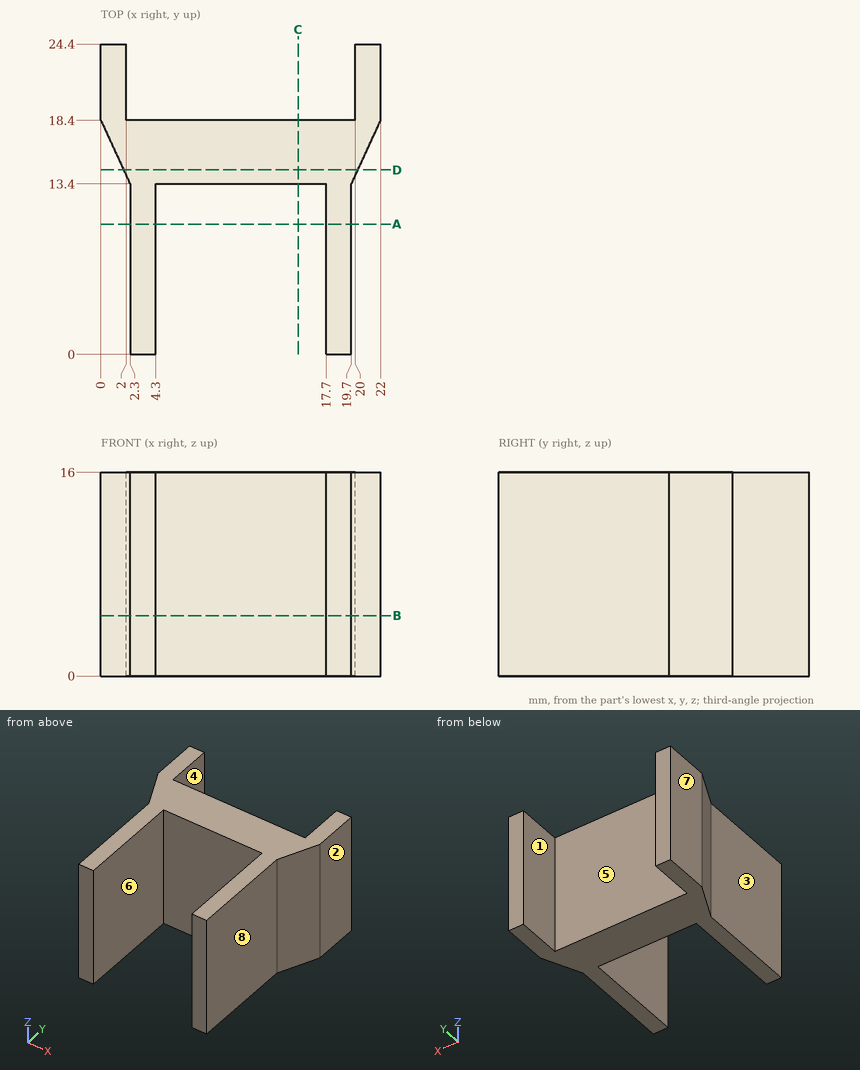
Answer from the drawing. Dimensions are ordinates in mm from the lowest x, y and z of the part. A direction names the side the tool comes from. Coordinates: 2 decimals unless noted, no trailing zeros. Write each loop counter-clockwise with the first axis right and the second up, starting at its lowest first coordinate (ties: lowest second). Pieces come first, ordered by that corner, then holes. Notation, with made-up numbers: M 11.5,-1.5 L 42.5,-1.5 A22 cw 42.5,13.5 Z; hole C -30.75,-36.5 d8. An arc over 180 degrees is marked long. Put each result on its own line as item: value. Start each with the question number.
1. Consider line 1 (X direction, y = 10.75, z = 4.5); line 2 (X direction, y = 23.25, z = 1); line 3 (Y direction, x = 2.5, z = 1.75). Determine where each line is inside the solid, lowest interval first. Write a range as from..to.
2. Which of the six approach directions +Z, -Z, +X, -X, +Y, -Y give full straight-line access (tool end or side, diameter ignored) to the marked faces 5, 6, 7 and 8?
3. A cutting plane is placed at B-B on z = 4.75. Write down the section's boundary in (x, y), then the cut area to 3 significant figures.
4. For a pull along X with two mould halves and no side action, classify the marked faces 1, 2, 3 and 4 as pulls with the +X half, pulls with the -X half, needs draft (parallel to the pull), parting line crosses it, or undercut.
5. A cutting plane is placed at D-D on y = 14.5. Write down the section's boundary in (x, z).
6. Flat-ended cylindrical pins translate along their axes: P1, Ø8, axis at x = 14.5, z = 11, coming from the +Y side; P2, Ø3, axis at y = 4, z = 6.5, coming from the +X side; P3, Ø8, axis at y = 6.5, z = 14, coming from the -X side. Find the tip coordinate at first contact, or state that the pin passes through.
7. A cutting plane is placed at A-A on y = 10.25. Write down the section's boundary in (x, z), then the cut area to 3 significant figures.
8. A cutting plane is placed at C-C on x = 15.5. Write down the section's boundary in (y, z).
Resolved:
1. line 1: x = 2.3..4.3, 17.7..19.7
1. line 2: x = 0..2, 20..22
1. line 3: y = 0..18.4
2. face 5: +Z, -Z, +Y
2. face 6: +Z, -Z, -Y
2. face 7: +Z, -Z, -X, +Y, -Y
2. face 8: +Z, -Z, +X, -Y
3. outline: M 0,18.4 L 2.3,13.4 L 2.3,0 L 4.3,0 L 4.3,13.4 L 17.7,13.4 L 17.7,0 L 19.7,0 L 19.7,13.4 L 22,18.4 L 22,24.4 L 20,24.4 L 20,18.4 L 2,18.4 L 2,24.4 L 0,24.4 Z
3. area: 176 mm2
4. face 1: undercut
4. face 2: pulls with the +X half
4. face 3: pulls with the -X half
4. face 4: undercut
5. outline: M 1.79,0 L 20.21,0 L 20.21,16 L 1.79,16 Z
6. P1: stops at y = 18.4
6. P2: stops at x = 19.7
6. P3: stops at x = 2.3
7. outline: M 2.3,0 L 4.3,0 L 4.3,16 L 2.3,16 Z; M 17.7,0 L 19.7,0 L 19.7,16 L 17.7,16 Z
7. area: 64.0 mm2
8. outline: M 13.4,0 L 18.4,0 L 18.4,16 L 13.4,16 Z
